```python
from build123d import *

# Parameters (mm, degrees)
BOSS_EXTRUDE1_DEPTH = 10
SKETCH3_R           = 2.25
CUT_EXTRUDE1_DEPTH  = 208.932080257
CIRPATTERN1_COUNT   = 3
CIRPATTERN1_ANGLE   = 30
CHAMFER1_SIZE       = 2


with BuildPart() as part:
    # Sketch2 → Boss-Extrude1 (new body)
    with BuildSketch(Plane(origin=(0, 0, 0), x_dir=(1, 0, 0), z_dir=(0, 1, 0))):
        with BuildLine():
            Line((-157, 0), (-147, 0))
            ThreePointArc((-147, 0), (-127.305734356, 73.5), (-73.5, 127.305734356))
            Line((-73.5, 127.305734356), (-78.5, 135.965988394))
            ThreePointArc((-78.5, 135.965988394), (-135.965988394, 78.5), (-157, 0))
        make_face()
    extrude(amount=BOSS_EXTRUDE1_DEPTH)

    # Sketch3 → Cut-Extrude1 (cut, through all)
    with BuildSketch(Plane(origin=(0, 10, 0), x_dir=(1, 0, 0), z_dir=(0, 1, 0))):
        with Locations(Location((-146.820725596, 39.340494856, 0), (0, 0, 270))):
            Circle(SKETCH3_R)
    cut_extrude1 = extrude(amount=-CUT_EXTRUDE1_DEPTH, mode=Mode.SUBTRACT)

    # CirPattern1: Cut-Extrude1 ×3 about axis
    cirpattern1_axis = Axis((0, 0, 0), (0, -1, 0))
    for i in range(1, CIRPATTERN1_COUNT):
        add(cut_extrude1.rotate(cirpattern1_axis, i * CIRPATTERN1_ANGLE / (CIRPATTERN1_COUNT - 1)), mode=Mode.SUBTRACT)

    # Chamfer1
    chamfer1_edges = [part.edges().sort_by_distance(p)[0] for p in [
        (-152, 10, 0),
        (-127.305734356, 10, -73.5),
        (-76, 10, -131.635861375),
    ]]
    chamfer(chamfer1_edges, length=CHAMFER1_SIZE)


solid = part.part
```
The model under review builds one solid part; all positions refer to its coordinate system, in mm. Round coordinates to 2 decimals unless told otherwise and drop trailing zeros. Loops run counter-clockwise (first coordinate to the right, second up) from the corner with the lowest first, then second, coordinate; pieces in that order, holes last. Notation, with made-up numbers: M 38.25,44 L 73.25,44 A22 cw 73.25,65 Z; hole C 84.25,31 d11. An arc over 180 degrees is marked long. Answer as a JSON object with one key per item and string values.
(1) Draft analysis for pull direction Z (two halves, no side actions). For faces 1 (the flat face through (-128, 0, -73)), 2 (the cylindrical face through (-107.77, 5.07, -109.71)), 3 (the flat face through (-76.82, 8.99, -131.08)), state which applies: released by +Z, released by -Z, zero draft, split by the parting line, or undercut.
Resolved:
{"face 1": "zero draft", "face 2": "undercut", "face 3": "released by -Z"}
(2) Clearance check with flat-ended pins moving along their axes: P1, Ø1.5, axis at x = -103, y = 6, coming from the -Z side; P2, Ø1, axis at x = -108, y = 1, coming from the +Z side; P3, Ø1.5, axis at y = 4, z = -63, coming from the +X side; P4, Ø3.5, axis at x = -146.82, z = -39.34, coming from the -Y side. State where each tip first meets the part, or that it passes through.
Resolved:
{"P1": "z = -119.14", "P2": "z = -99.18", "P3": "x = -132.46", "P4": "through"}
(3) Take a section at A-A on y = 6.5. Give the boundary of the cut face in (x, z).
Resolved:
{"outline": "M -157,0 A157 ccw -78.5,-135.97 L -73.5,-127.31 A147 cw -147,0 Z; hole C -146.82,-39.34 d4.5; hole C -131.64,-76 d4.5; hole C -107.48,-107.48 d4.5"}
(4) To check wall thickness, follow line 1 along Z through (x, y) = (-106.5, 0.75); line 2 along X through (y, z) = (9.75, -108.5); line 3 along Z through (x, y) = (-132.5, 2). State the ranges of each line that lie inside material, in increasing order.
Resolved:
{"line 1": "-115.35 to -109.51, -105.45 to -101.32", "line 2": "-113.48 to -109.49, -105.47 to -101.76", "line 3": "-84.22 to -78.08, -73.92 to -63.66"}
